from build123d import *

# Parameters (mm, degrees)
F0_R     = 4
F1_DEPTH = 30
F2_R     = 2
F3_DEPTH = 25
F4_R     = 4.5
F5_DEPTH = 1.5
F6_R     = 4.5
F7_DEPTH = 1.5
F8_R     = 1


with BuildPart() as f1:
    # F0 (on Front) → F1 (new body)
    with BuildSketch(Plane.XZ):
        Polygon((-10, 5), (-17, 5), (-17, -12), (17, -12), (17, 5), (10, 5), (5, 8), (-5, 8), align=None)
        Circle(F0_R, mode=Mode.SUBTRACT)
    extrude(amount=F1_DEPTH)

    # F2 (on face) → F3 (cut)
    with BuildSketch(Plane(origin=(0, 0, -12), x_dir=(1, 0, 0), z_dir=(0, 0, -1))):
        with Locations((-13, 26)):
            Circle(F2_R)
        with Locations((-13, 4)):
            Circle(F2_R)
        with Locations((13, 26)):
            Circle(F2_R)
        with Locations((13, 4)):
            Circle(F2_R)
    extrude(amount=-F3_DEPTH, mode=Mode.SUBTRACT)

    # F4 (on face) → F5 (cut)
    with BuildSketch(Plane.XZ.offset(30)):
        Circle(F4_R)
    extrude(amount=-F5_DEPTH, mode=Mode.SUBTRACT)

    # F6 (on face) → F7 (cut)
    with BuildSketch(Plane(origin=(0, 0, 0), x_dir=(-1, 0, 0), z_dir=(0, 1, 0))):
        Circle(F6_R)
    extrude(amount=-F7_DEPTH, mode=Mode.SUBTRACT)

    # F8
    f8_edges = [f1.edges().sort_by_distance(p)[0] for p in [
        (-17, -15, 5),
        (-10, -15, 5),
        (-5, -15, 8),
        (5, -15, 8),
        (10, -15, 5),
        (17, -15, 5),
    ]]
    fillet(f8_edges, radius=F8_R)


solid = f1.part
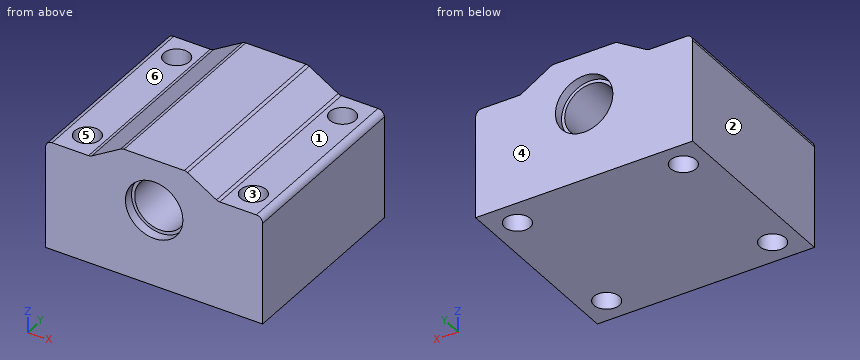
Design review of the part built by this model. Coordinates are the model's own, in mm. Face numbers are marked on the shaded views. A direction names the side the tool comes from. Coordinates: 2 decimals unless noted, no trailing zeros. Write each loop counter-clockwise with the first axis right and the second up, starting at its lowest first coordinate (ties: lowest second). Pieces come first, ordered by that corner, then holes. Notation, with made-up numbers: (19.5, 23.25) -> (47.5, 23.25) arc R27 cw to (47.5, 48.25) -> close; hole circle Ø2 at (74, 15.5). An arc over 180 degrees is marked (long way). Write each question's results on one line, items separated by ' | '. Start each with the question number.
(1) Take a section at C-C on x = 0. Write out the cut boundary in (y, z).
(2) Take a section at B-B on z = 0. Write out the cut boundary in (x, y), and give its area (3 significant figures).
(3) The part is to be moulded in two halves that separate along Y. For the marked faces 3, 4, 5 and 6, say which applies: pulls with the +Y half, pulls with the -Y half, needs draft (parallel to the pull), parting line crosses it, or undercut.
(4) Take a section at D-D on y = -17. Write out the cut boundary in (x, z), and give its area (3 significant figures).
(5) Take a section at A-A on y = -4. Write out the cut boundary in (x, z), and give its area (3 significant figures).
(6) For line 1 along Y through (x, z) = (13, 1.25); line 2 along X through (y, z) = (-26, -6.5); line 3 along Y through (x, z) = (12, -2.5), list the stretches that pass through material, from the lowest coordinate up. Write a range as from..to.
(7) Clearance check with flat-ended pins moving along their axes: P1, Ø3.5, axis at x = 13, y = -4, coming from the -Z side; P2, Ø4.5, axis at x = -13, y = -4, coming from the +Z side; P3, Ø5, axis at x = -12, y = -6.5, coming from the +Z side; P4, Ø6, axis at x = -9.5, y = -13, coming from the +Z side. State where each tip first meets the part, or that it passes through.
(8) Tool access review of the marked faces 1 and 2: name each direction out of +Z, -Z, +X, -X, +Y, -Y from which nothing blocks a thin tool from reaching the whole face with its end or side.
Results found:
1) outline: (-30, -12) -> (0, -12) -> (0, -4.5) -> (-1.5, -4.5) -> (-1.5, -4) -> (-28.5, -4) -> (-28.5, -4.5) -> (-30, -4.5) -> close; (-30, 4.5) -> (-28.5, 4.5) -> (-28.5, 4) -> (-1.5, 4) -> (-1.5, 4.5) -> (0, 4.5) -> (0, 8) -> (-30, 8) -> close
2) outline: (-17, -30) -> (-4.5, -30) -> (-4.5, -28.5) -> (-4, -28.5) -> (-4, -1.5) -> (-4.5, -1.5) -> (-4.5, 0) -> (-17, 0) -> close; (4, -28.5) -> (4.5, -28.5) -> (4.5, -30) -> (17, -30) -> (17, 0) -> (4.5, 0) -> (4.5, -1.5) -> (4, -1.5) -> close; hole circle Ø4 at (-13, -26); hole circle Ø4 at (-13, -4); hole circle Ø4 at (13, -26); hole circle Ø4 at (13, -4) | area: 727 mm2
3) face 3: undercut | face 4: pulls with the +Y half | face 5: undercut | face 6: needs draft
4) outline: (-17, -12) -> (17, -12) -> (17, 4) arc R1 ccw to (16, 5) -> (10.28, 5) arc R1 cw to (9.76, 5.14) -> (5.24, 7.86) arc R1 ccw to (4.72, 8) -> (-4.72, 8) arc R1 ccw to (-5.24, 7.86) -> (-9.76, 5.14) arc R1 cw to (-10.28, 5) -> (-16, 5) arc R1 ccw to (-17, 4) -> close; hole circle Ø8 at (0, 0) | area: 572 mm2
5) outline: (-17, -12) -> (-15, -12) -> (-15, 5) -> (-16, 5) arc R1 ccw to (-17, 4) -> close; (-11, -12) -> (11, -12) -> (11, 5) -> (10.28, 5) arc R1 cw to (9.76, 5.14) -> (5.24, 7.86) arc R1 ccw to (4.72, 8) -> (-4.72, 8) arc R1 ccw to (-5.24, 7.86) -> (-9.76, 5.14) arc R1 cw to (-10.28, 5) -> (-11, 5) -> close; (15, -12) -> (17, -12) -> (17, 4) arc R1 ccw to (16, 5) -> (15, 5) -> close; hole circle Ø8 at (0, 0) | area: 436 mm2
6) line 1: y = -30..-28, -24..-6, -2..0 | line 2: x = -17..-15, -11..11, 15..17 | line 3: y = -30..-27.73, -24.27..-5.73, -2.27..0
7) P1: passes through | P2: stops at z = 5 | P3: stops at z = 5.3 | P4: stops at z = 7.1
8) face 1: +Z, +X, +Y, -Y | face 2: +Z, -Z, -X, +Y, -Y
